```python
from build123d import *

# Parameters (mm, degrees)
SKETCH_3_W          = 90
SKETCH_3_H          = 120
SKETCH_3_R          = 2
EXTRUDE_2_DEPTH     = 7
FILLET_1_R          = 5
FILLET_2_R          = 5
FILLET_3_R          = 5
FILLET_4_R          = 5
FILLET_5_R          = 5
FILLET_6_R          = 5
SKETCH_4_W          = 9.2
SKETCH_4_H          = 3.3
CUT_EXTRUDE_1_DEPTH = 3
FILLET_7_R          = 0.5
FILLET_8_R          = 0.5
FILLET_9_R          = 0.5
FILLET_10_R         = 0.5
SKETCH_5_R          = 2.058488494
CUT_EXTRUDE_2_DEPTH = 3


with BuildPart() as part:
    # 草图3 → 凸台-拉伸2 (new body)
    with BuildSketch(Plane(origin=(0, 0, 0), x_dir=(-1, 0, 0), z_dir=(0, 1, 0))):
        Rectangle(SKETCH_3_W, SKETCH_3_H)
        with Locations(Location((40, 55, 0), (0, 0, 90))):
            Circle(SKETCH_3_R, mode=Mode.SUBTRACT)
        with Locations(Location((40, -55, 0), (0, 0, 90))):
            Circle(SKETCH_3_R, mode=Mode.SUBTRACT)
        with Locations(Location((-40, -55, 0), (0, 0, 90))):
            Circle(SKETCH_3_R, mode=Mode.SUBTRACT)
        with Locations(Location((-40, 55, 0), (0, 0, 90))):
            Circle(SKETCH_3_R, mode=Mode.SUBTRACT)
        Polygon((-42, -50), (-42, 50), (-35, 50), (-35, 57), (35, 57), (35, 50), (42, 50), (42, -50), (35, -50), (35, -57), (-35, -57), (-35, -50), align=None, mode=Mode.SUBTRACT)
    extrude(amount=EXTRUDE_2_DEPTH)

    # 圆角1
    fillet_1_edges = [part.edges().sort_by_distance(p)[0] for p in [
        (45, 3.5, -60),
        (45, 3.5, 60),
        (-45, 3.5, 60),
    ]]
    fillet(fillet_1_edges, radius=FILLET_1_R)

    # 圆角2
    fillet_2_edges = [part.edges().sort_by_distance(p)[0] for p in [
        (-45, 3.5, -60),
    ]]
    fillet(fillet_2_edges, radius=FILLET_2_R)

    # 圆角3
    fillet_3_edges = [part.edges().sort_by_distance(p)[0] for p in [
        (35, 3.5, -50),
    ]]
    fillet(fillet_3_edges, radius=FILLET_3_R)

    # 圆角4
    fillet_4_edges = [part.edges().sort_by_distance(p)[0] for p in [
        (-35, 3.5, -50),
    ]]
    fillet(fillet_4_edges, radius=FILLET_4_R)

    # 圆角5
    fillet_5_edges = [part.edges().sort_by_distance(p)[0] for p in [
        (35, 3.5, 50),
    ]]
    fillet(fillet_5_edges, radius=FILLET_5_R)

    # 圆角6
    fillet_6_edges = [part.edges().sort_by_distance(p)[0] for p in [
        (-35, 3.5, 50),
    ]]
    fillet(fillet_6_edges, radius=FILLET_6_R)

    # 草图4 → 切除-拉伸1 (cut)
    with BuildSketch(Plane(origin=(0, 0, -60), x_dir=(-1, 0, 0), z_dir=(0, 0, -1))):
        with Locations((-26.1, 2.65)):
            Rectangle(SKETCH_4_W, SKETCH_4_H)
    extrude(amount=-CUT_EXTRUDE_1_DEPTH, mode=Mode.SUBTRACT)

    # 圆角7
    fillet_7_edges = [part.edges().sort_by_distance(p)[0] for p in [
        (21.5, 1, -58.5),
    ]]
    fillet(fillet_7_edges, radius=FILLET_7_R)

    # 圆角8
    fillet_8_edges = [part.edges().sort_by_distance(p)[0] for p in [
        (21.5, 4.3, -58.5),
    ]]
    fillet(fillet_8_edges, radius=FILLET_8_R)

    # 圆角9
    fillet_9_edges = [part.edges().sort_by_distance(p)[0] for p in [
        (30.7, 1, -58.5),
    ]]
    fillet(fillet_9_edges, radius=FILLET_9_R)

    # 圆角10
    fillet_10_edges = [part.edges().sort_by_distance(p)[0] for p in [
        (30.7, 4.3, -58.5),
    ]]
    fillet(fillet_10_edges, radius=FILLET_10_R)

    # 草图5 → 切除-拉伸2 (cut)
    with BuildSketch(Plane(origin=(0, 0, -60), x_dir=(-1, 0, 0), z_dir=(0, 0, -1))):
        with Locations((-16.5, 2.913308791)):
            Circle(SKETCH_5_R)
    extrude(amount=-CUT_EXTRUDE_2_DEPTH, mode=Mode.SUBTRACT)


solid = part.part
```
Geometry: final body of the model. Coordinates: model frame, mm. A direction names the side the tool comes from. Round coordinates to 2 decimals unless told otherwise and drop trailing zeros. Write each loop counter-clockwise with the first axis right and the second up, starting at its lowest first coordinate (ties: lowest second). Pieces come first, ordered by that corner, then holes.
Item 1: Section query B-B (x = 25). Return loops of the section in (y, z), plus the area to 3 significant figures.
Item 2: Section query C-C (x = -8). Return loops of the section in (y, z).
Item 3: Pin query (flat end, axial travel): P1, Ø2.5, axis at x = -40, z = -55, coming from the -Y side; P2, Ø2, axis at x = -41.5, y = 2, coming from the -Z side; P3, Ø0.6, axis at y = 2.5, z = -56, coming from the -X side; P4, Ø1.8, axis at y = 2.5, z = -58.5, coming from the -X side. Return the tip coordinate at first contact, or that it passes through.
Item 4: Section query A-A (z = 18.5). Return loops of the section in (x, y).
Item 5: Material intervals for L1, parallel to X at y = 4.5, z = -55; L2, parallel to Z at x = -24.5, y = 2.25; L3, parallel to X at y = 0.75, z = 34, sorted ascending.
Item 6: Set-up query: faces 1 (the face through (-43, 4, 59)), 2 (the face through (-42, 3, 1)), 3 (the face through (18.134, 1.661, -58.521)). Return all of +Z, -Z, +X, -X, +Y, -Y with unobstructed straight access to the full face (end or side cutting, diameter ignored); none if empty.
Item 7: Mould query, pull axis X, two halves, no side actions, for faces 4 (the face through (45, 3, -1)), 5 (the face through (1, 3, -60)), 6 (the face through (-43, 4, -59)), 7 (the face through (37, 4, -51)). Classes: +X half, -X half, draft (parallel to the pull), parting line (faces both ways), or undercut.
Completed:
1. outline: (0, -60) - (1, -60) - (1, -57) - (0, -57) - close; (0, 57) - (7, 57) - (7, 60) - (0, 60) - close; (4.3, -60) - (7, -60) - (7, -57) - (4.3, -57) - close
1. area: 32.1 mm2
2. outline: (0, -60) - (7, -60) - (7, -57) - (0, -57) - close; (0, 57) - (7, 57) - (7, 60) - (0, 60) - close
3. P1: passes through
3. P2: stops at z = -59.97
3. P3: stops at x = -44.95
3. P4: stops at x = -44.27
4. outline: (-45, 0) - (-42, 0) - (-42, 7) - (-45, 7) - close; (42, 0) - (45, 0) - (45, 7) - (42, 7) - close
5. L1: x = -45 to -42, -38 to -35, 35 to 38, 42 to 45
5. L2: z = -60 to -57, 57 to 60
5. L3: x = -45 to -42, 42 to 45
6. face 1: +Z, -X, +Y, -Y
6. face 2: +Y, -Y
6. face 3: -Z
7. face 4: +X half
7. face 5: draft
7. face 6: -X half
7. face 7: undercut
